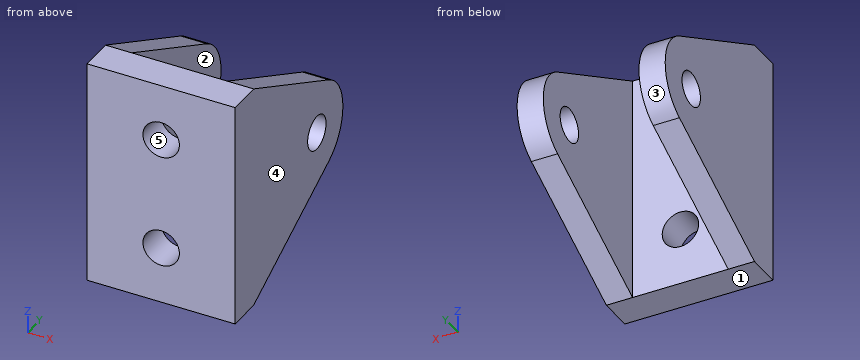
from build123d import *

# Parameters (mm, degrees)
SKETCH_1_W          = 13
SKETCH_1_H          = 20
SKETCH_1_R          = 1.6
EXTRUDE_1_DEPTH     = 3
SKETCH_2_R          = 1.5
EXTRUDE_2_DEPTH     = 13
SKETCH_3_W          = 8.4
SKETCH_3_H          = 14.54
CUT_EXTRUDE_1_DEPTH = 28.384331286


with BuildPart() as part:
    # 草图1 → 凸台-拉伸1 (new body)
    with BuildSketch(Plane(origin=(0, 0, 0), x_dir=(1, 0, 0), z_dir=(0, 1, 0))):
        Rectangle(SKETCH_1_W, SKETCH_1_H)
        with Locations(Location((0, 5, 0), (0, 0, 270))):
            Circle(SKETCH_1_R, mode=Mode.SUBTRACT)
        with Locations(Location((0, -5, 0), (0, 0, 90))):
            Circle(SKETCH_1_R, mode=Mode.SUBTRACT)
    extrude(amount=EXTRUDE_1_DEPTH)

    # 草图2 → 凸台-拉伸2 (add)
    with BuildSketch(Plane.ZY.offset(6.5)):
        with BuildLine():
            Line((-10, 3), (10, 3))
            Line((10, 3), (3.778714502, 15.223256798))
            ThreePointArc((3.778714502, 15.223256798), (0, 17.54), (-3.778714502, 15.223256798))
            Line((-3.778714502, 15.223256798), (-10, 3))
        make_face()
        with Locations((0, 13.3)):
            Circle(SKETCH_2_R, mode=Mode.SUBTRACT)
    extrude(amount=-EXTRUDE_2_DEPTH)

    # 草图3 → 切除-拉伸1 (cut, through all)
    with BuildSketch(Plane(origin=(0, 0, -10), x_dir=(-1, 0, 0), z_dir=(0, 0, -1))):
        with Locations((0, 10.27)):
            Rectangle(SKETCH_3_W, SKETCH_3_H)
    extrude(amount=-CUT_EXTRUDE_1_DEPTH, mode=Mode.SUBTRACT)


solid = part.part
Check sheet for the modelled part. Datum: model origin and axes. Units: mm. Face numbers are marked on the shaded views. A direction names the side the tool comes from. Give positions to 0.01 mm unless a question says otherwise; leave off trailing zeros. Loops run counter-clockwise (first coordinate to the right, second up) from the corner with the lowest first, then second, coordinate; pieces in that order, holes last. Notation, with made-up numbers: M 56.5,83.25 L 101.5,83.25 A34 cw 101.5,114.25 Z; hole C 70,36.5 d1. An arc over 180 degrees is marked long. Return JSON: item names as keys, results as strings. Group by question number.
1. Thickness scan on L1, parallel to X at y = 1.35, z = -5; L2, parallel to X at y = 14.75, z = -3.75; L3, parallel to Y at x = 1.25, z = 3. Record the ranges inside material, lowest first.
2. Go/stop test with flat-tipped pins: pin 1 (2.5 mm diameter, centred on y = 13.3, z = 0, fed in from +X); pin 2 (5 mm diameter, centred on x = 0, z = -6.5, fed in from +Y); pin 3 (6 mm diameter, centred on x = 4.5, y = 7, fed in from +Z). Record where each tip stops, or that it passes through.
3. Tool access check on the marked faces 1 and 2. Record the directions out of +Z, -Z, +X, -X, +Y, -Y that give a thin tool (end or side, any length) a straight path to the whole face; none if there is none.
4. Cross-section at C-C on x = 0. Record the boundary of the cut face in (y, z), plus the area to 3 significant figures.
5. Mould release check, pull along X, two halves, no side actions. Record for the marked faces 3, 4 and 5: released by +X, released by -X, zero draft, split by the parting line, or undercut.
6. Cross-section at A-A on x = 5.25. Record the boundary of the cut face in (y, z).
7. Cross-section at D-D on z = -5. Record the boundary of the cut face in (x, y), plus the area to 3 significant figures.
8. Cross-section at B-B on y = 5.5. Record the boundary of the cut face in (x, z).
Return value:
{
 "1": {"L1": "-6.5 to -1.6, 1.6 to 6.5", "L2": "-6.5 to -4.2, 4.2 to 6.5", "L3": "0 to 3"},
 "2": {"pin 1": "through", "pin 2": "y = 3", "pin 3": "z = 9.49"},
 "3": {"face 1": "-Z, +X, -X, +Y, -Y", "face 2": "+Z, -Z, +Y"},
 "4": {"outline": "M 0,-10 L 3,-10 L 3,-6.6 L 0,-6.6 Z; M 0,-3.4 L 3,-3.4 L 3,3.4 L 0,3.4 Z; M 0,6.6 L 3,6.6 L 3,10 L 0,10 Z", "area": "40.8 mm^2"},
 "5": {"face 3": "zero draft", "face 4": "released by +X", "face 5": "undercut"},
 "6": {"outline": "M 0,-10 L 3,-10 L 15.22,-3.78 A4.24 ccw 15.22,3.78 L 3,10 L 0,10 Z; hole C 13.3,0 d3"},
 "7": {"outline": "M -6.5,0 L -1.6,0 L -1.6,3 L -4.2,3 L -4.2,12.82 L -6.5,12.82 Z; M 1.6,0 L 6.5,0 L 6.5,12.82 L 4.2,12.82 L 4.2,3 L 1.6,3 Z", "area": "74.6 mm^2"},
 "8": {"outline": "M -6.5,-8.73 L -4.2,-8.73 L -4.2,8.73 L -6.5,8.73 Z; M 4.2,-8.73 L 6.5,-8.73 L 6.5,8.73 L 4.2,8.73 Z"}
}
